Autodesk Inventor part; units mm, degrees
ref_plane "YZ Plane" through (0, 0, 0) normal (1, 0, 0) x (0, 1, 0)
ref_plane "XZ Plane" through (0, 0, 0) normal (0, 1, 0) x (-1, 0, 0)
ref_plane "XY Plane" through (0, 0, 0) normal (0, 0, 1) x (1, 0, 0)
sketch "Sketch1" plane through (0, 0, 0) normal (0, 1, 0) x (-1, 0, 0)
  line L0 (0, 0) -> (45, 0)
  line L1 (45, 0) -> (14.87, 0)
  line L2 (14.87, -170.18) -> (56.523, -170.18)
  line L3 (144.78, -163.83) -> (144.78, -85.18)
  line L4 (144.78, -85.18) -> (45, -85.18)
  line L5 (144.78, -163.83) -> (144.78, -170.18)
  line L6 (113.657, -170.18) -> (144.78, -170.18)
  line L7 (144.78, -170.18) -> (0, -170.18)
  line L8 (45, 0) -> (45, -85.18)
  circle A0 centre (5.08, -6.35) radius 1.75
  circle A1 centre (5.08, -163.83) radius 1.75
  circle A2 centre (137.16, -163.83) radius 1.75
  circle A3 centre (83.48, -93.35) radius 1.75
  circle A4 centre (83.48, -156.35) radius 1.75
  line L9 (-36.027, -96.0808) -> (-36.027, -97.5854)
  line L10 (-39.0316, -99.0854) -> (-39.0316, -71.0946)
  line L11 (-8.0362, -74.0992) -> (-8.0362, -72.5946)
  line L12 (-8.0362, -72.5946) -> (-8.0362, -74.0992)
  line L13 (-36.027, -68.09) -> (-8.0362, -68.09)
  arc A5 (-36.027, -96.0808) -> (-39.0316, -99.0854) centre (-36.027, -99.0854) ccw
  arc A6 (-8.0362, -68.09) -> (-11.0408, -71.0946) centre (-8.0362, -71.0946) ccw
  arc A7 (-36.027, -97.5854) -> (-34.527, -99.0854) centre (-36.027, -99.0854) ccw
  arc A8 (-36.027, -97.5854) -> (-34.527, -99.0854) centre (-36.027, -99.0854) ccw
  arc A9 (-8.0362, -72.5946) -> (-9.5362, -71.0946) centre (-8.0362, -71.0946) ccw
  arc A10 (-8.0362, -72.5946) -> (-9.5362, -71.0946) centre (-8.0362, -71.0946) ccw
  arc A11 (-8.0362, -74.0992) -> (-5.0316, -71.0946) centre (-8.0362, -71.0946) ccw
  line L14 (-5.0316, -99.0854) -> (-5.0316, -71.0946)
  line L15 (-8.0362, -102.09) -> (-36.027, -102.09)
  line L16 (-36.027, -102.09) -> (-8.0362, -102.09)
  arc A12 (-9.5362, -99.0854) -> (-8.0362, -97.5854) centre (-8.0362, -99.0854) ccw
  arc A13 (-9.5362, -99.0854) -> (-8.0362, -97.5854) centre (-8.0362, -99.0854) ccw
  arc A14 (-34.527, -71.0946) -> (-36.027, -72.5946) centre (-36.027, -71.0946) ccw
  arc A15 (-34.527, -71.0946) -> (-36.027, -72.5946) centre (-36.027, -71.0946) ccw
  line L17 (-8.0362, -97.5854) -> (-8.0362, -96.0808)
  arc A16 (-5.0316, -99.0854) -> (-8.0362, -96.0808) centre (-8.0362, -99.0854) ccw
  arc A17 (-5.0316, -99.0854) -> (-8.0362, -96.0808) centre (-8.0362, -99.0854) ccw
  line L18 (-8.0362, -97.5854) -> (-8.0362, -96.0808)
  line L19 (-34.527, -71.0946) -> (-33.0224, -71.0946)
  arc A18 (-33.0224, -71.0946) -> (-36.027, -68.09) centre (-36.027, -71.0946) ccw
  arc A19 (-39.0316, -71.0946) -> (-36.027, -74.0992) centre (-36.027, -71.0946) ccw
  arc A20 (-39.0316, -71.0946) -> (-36.027, -74.0992) centre (-36.027, -71.0946) ccw
  arc A21 (-33.0224, -71.0946) -> (-36.027, -68.09) centre (-36.027, -71.0946) ccw
  line L20 (-11.0408, -71.0946) -> (-9.5362, -71.0946)
  line L21 (-9.5362, -71.0946) -> (-11.0408, -71.0946)
  line L22 (-36.027, -97.5854) -> (-36.027, -96.0808)
  arc A22 (-36.027, -96.0808) -> (-39.0316, -99.0854) centre (-36.027, -99.0854) ccw
  line L23 (-34.527, -99.0854) -> (-33.0224, -99.0854)
  line L24 (-34.527, -99.0854) -> (-33.0224, -99.0854)
  arc A23 (-36.027, -102.09) -> (-33.0224, -99.0854) centre (-36.027, -99.0854) ccw
  line L25 (-11.0408, -99.0854) -> (-9.5362, -99.0854)
  line L26 (-11.0408, -99.0854) -> (-9.5362, -99.0854)
  arc A24 (-11.0408, -99.0854) -> (-8.0362, -102.09) centre (-8.0362, -99.0854) ccw
  line L27 (-36.027, -74.0992) -> (-36.027, -72.5946)
  line L28 (-36.027, -72.5946) -> (-36.027, -74.0992)
  line L29 (-36.027, -99.0854) -> (-23.327, -99.0854) construction
  line L30 (-36.027, -99.0854) -> (-27.137, -99.0854) construction
  arc A25 (-44.0632, -105.3716) -> (-42.3132, -107.1216) centre (-42.3132, -105.3716) ccw
  arc A26 (-42.3132, -63.0584) -> (-44.0632, -64.8084) centre (-42.3132, -64.8084) ccw
  line L31 (-42.3132, -63.0584) -> (0, -63.0584)
  line L32 (0, -107.1216) -> (-42.3132, -107.1216)
  line L33 (-44.0632, -105.3716) -> (-44.0632, -64.8084)
  line L34 (0, -170.18) -> (0, -107.1216)
  line L35 (0, -63.0584) -> (0, 0)
  circle A27 centre (10.16, -127.8558) radius 1.5
  circle A28 centre (10.16, -149.4458) radius 1.5
  circle A29 centre (25.4, -149.4458) radius 1.5
  circle A30 centre (25.4, -127.8558) radius 1.4986
  point P0 (-2.54, 0.1)
  dimension "d3" = 3.5
  dimension "d5" = 3.5
  dimension "d6" = 3.5
  dimension "d9" = 3
  dimension "d10" = 3
  dimension "d11" = 3
  dimension "d12" = 2.9972
extrude "Extrusion1" add sketch "Sketch1" along normal blind 2.286
fillet "Fillet1" radius 3.175 8 edges at (-45, 1.143, 0) (0, 1.143, 0) (0, 1.143, -63.0584) (0, 1.143, -107.1216) (-45, 1.143, -85.18) (-144.78, 1.143, -85.18) (-144.78, 1.143, -170.18) (0, 1.143, -170.18)
sketch "Sketch2" plane through (0, 2.286, 0) normal (0, 1, 0) x (1, 0, 0)
  circle A0 centre (-51.7938, 156.5362) radius 1.75
  circle A1 centre (-115.1662, 156.5362) radius 1.75
  circle A2 centre (-115.1662, 93.1638) radius 1.65
  circle A3 centre (-115.1662, 93.1638) radius 1.75
  circle A4 centre (-51.7938, 93.1638) radius 1.65
  circle A5 centre (-51.7938, 93.1638) radius 1.75
  line L0 (-144.78, 167.005) -> (-144.78, 88.355)
  line L1 (0, 110.2966) -> (0, 167.005)
  circle A6 centre (-83.48, 93.35) radius 1.75
  circle A7 centre (-83.48, 156.35) radius 1.75
  point P0 (0, 0)
  dimension "d17" = 3.5
  dimension "d18" = 3.5
  dimension "d19" = 3.5
  dimension "d20" = 3.5
extrude "Extrusion2" cut sketch "Sketch2" against normal blind 25.4 contours A0 | A1 | A2 | A3 | A4 | A5
sketch "Sketch3" plane through (0, 2.286, 0) normal (0, 1, 0) x (1, 0, 0)
  circle A0 centre (-5.08, 6.35) radius 1.75
  arc A1 (-17.78, 9.525) -> (-11.43, 9.525) centre (-14.605, 9.525) ccw
  arc A2 (-30.48, 9.525) -> (-24.13, 9.525) centre (-27.305, 9.525) ccw
  arc A3 (-11.43, 73.025) -> (-17.78, 73.025) centre (-14.605, 73.025) ccw
  arc A4 (-24.13, 98.425) -> (-30.48, 98.425) centre (-27.305, 98.425) ccw
  line L0 (-30.48, 9.525) -> (-30.48, 98.425)
  line L1 (-24.13, 98.425) -> (-24.13, 9.525)
  line L2 (-17.78, 9.525) -> (-17.78, 73.025)
  line L3 (-11.43, 73.025) -> (-11.43, 9.525)
  point P0 (0, 0)
extrude "Extrusion3" cut sketch "Sketch3" against normal blind 25.4 contours L2 A3 L3 A1 | L0 A4 L1 A2
sketch "Sketch4" plane through (0, 2.286, 0) normal (0, 1, 0) x (1, 0, 0)
  circle A0 centre (-5.08, 6.35) radius 1.75
  circle A1 centre (-5.08, 6.35) radius 1.75
  arc A2 (-5.08, 11.43) -> (-5.08, 1.27) centre (-5.08, 6.35) ccw
  line L0 (0, 3.175) -> (0, 59.8834)
  line L1 (-5.08, 1.27) -> (5.0316, 1.27)
  line L2 (5.0316, 1.27) -> (5.0316, 63.0584)
  line L3 (-5.08, 11.43) -> (0, 11.43)
  line L4 (0, 11.43) -> (0, 59.8834)
  line L5 (3.175, 63.0584) -> (42.3132, 63.0584)
  line L6 (5.0316, 63.0584) -> (42.3132, 63.0584)
  line L7 (44.0632, 64.8084) -> (44.0632, 105.3716)
  line L8 (44.0632, 64.8084) -> (44.0632, 105.3716)
  line L9 (42.3132, 107.1216) -> (3.175, 107.1216)
  line L10 (42.3132, 107.1216) -> (5.0316, 107.1216)
  line L11 (5.0316, 107.1216) -> (5.0316, 170.18)
  circle A3 centre (-5.08, 163.83) radius 1.75
  circle A4 centre (-5.08, 163.83) radius 1.75
  circle A5 centre (-5.08, 163.83) radius 5.08
  line L12 (0, 110.2966) -> (0, 167.005)
  line L13 (-5.08, 168.91) -> (5.0316, 168.91)
  line L14 (0, 59.8834) -> (0, 158.75)
  line L15 (0, 158.75) -> (-5.08, 158.75)
  arc A6 (8.0362, 72.5946) -> (9.5362, 71.0946) centre (8.0362, 71.0946) ccw
  arc A7 (8.0362, 72.5946) -> (9.5362, 71.0946) centre (8.0362, 71.0946) ccw
  arc A8 (34.527, 71.0946) -> (36.027, 72.5946) centre (36.027, 71.0946) ccw
  arc A9 (34.527, 71.0946) -> (36.027, 72.5946) centre (36.027, 71.0946) ccw
  arc A10 (36.027, 97.5854) -> (34.527, 99.0854) centre (36.027, 99.0854) ccw
  arc A11 (36.027, 97.5854) -> (34.527, 99.0854) centre (36.027, 99.0854) ccw
  arc A12 (9.5362, 99.0854) -> (8.0362, 97.5854) centre (8.0362, 99.0854) ccw
  arc A13 (9.5362, 99.0854) -> (8.0362, 97.5854) centre (8.0362, 99.0854) ccw
  arc A14 (8.0362, 68.09) -> (11.0408, 71.0946) centre (8.0362, 71.0946) ccw
  arc A15 (33.0224, 71.0946) -> (36.027, 68.09) centre (36.027, 71.0946) ccw
  line L16 (11.0408, 99.0854) -> (9.5362, 99.0854)
  line L17 (36.027, 68.09) -> (8.0362, 68.09)
  line L18 (8.0362, 68.09) -> (36.027, 68.09)
  line L19 (5.0316, 99.0854) -> (5.0316, 71.0946)
  line L20 (5.0316, 71.0946) -> (5.0316, 99.0854)
  line L21 (8.0362, 102.09) -> (36.027, 102.09)
  line L22 (8.0362, 102.09) -> (36.027, 102.09)
  line L23 (39.0316, 71.0946) -> (39.0316, 99.0854)
  line L24 (39.0316, 71.0946) -> (39.0316, 99.0854)
  line L25 (33.0224, 71.0946) -> (34.527, 71.0946)
  line L26 (34.527, 71.0946) -> (33.0224, 71.0946)
  line L27 (36.027, 72.5946) -> (36.027, 74.0992)
  line L28 (36.027, 72.5946) -> (36.027, 74.0992)
  line L29 (9.5362, 71.0946) -> (11.0408, 71.0946)
  line L30 (11.0408, 71.0946) -> (9.5362, 71.0946)
  line L31 (8.0362, 74.0992) -> (8.0362, 72.5946)
  line L32 (8.0362, 72.5946) -> (8.0362, 74.0992)
  line L33 (8.0362, 96.0808) -> (8.0362, 97.5854)
  line L34 (8.0362, 96.0808) -> (8.0362, 97.5854)
  arc A16 (11.0408, 99.0854) -> (8.0362, 102.09) centre (8.0362, 99.0854) ccw
  line L35 (9.5362, 99.0854) -> (11.0408, 99.0854)
  line L36 (36.027, 97.5854) -> (36.027, 96.0808)
  line L37 (36.027, 96.0808) -> (36.027, 97.5854)
  line L38 (33.0224, 99.0854) -> (34.527, 99.0854)
  line L39 (34.527, 99.0854) -> (33.0224, 99.0854)
  arc A17 (36.027, 96.0808) -> (39.0316, 99.0854) centre (36.027, 99.0854) ccw
  arc A18 (36.027, 102.09) -> (33.0224, 99.0854) centre (36.027, 99.0854) ccw
  arc A19 (33.0224, 71.0946) -> (36.027, 68.09) centre (36.027, 71.0946) ccw
  arc A20 (39.0316, 71.0946) -> (36.027, 74.0992) centre (36.027, 71.0946) ccw
  arc A21 (8.0362, 68.09) -> (11.0408, 71.0946) centre (8.0362, 71.0946) ccw
  arc A22 (8.0362, 74.0992) -> (5.0316, 71.0946) centre (8.0362, 71.0946) ccw
  arc A23 (11.0408, 99.0854) -> (8.0362, 102.09) centre (8.0362, 99.0854) ccw
  arc A24 (5.0316, 99.0854) -> (8.0362, 96.0808) centre (8.0362, 99.0854) ccw
  point P0 (0, 0)
  point P1 (3.175, 59.8834)
properties part number "ThirdLayer"
The listing builds one solid part. Answer for the finished solid, in the listing's coordinates (mm). Round coordinates to 2 decimals unless told otherwise and drop trailing zeros. Loops run counter-clockwise (first coordinate to the right, second up) from the corner with the lowest first, then second, coordinate; pieces in that order, holes last. Notation, with made-up numbers: M 88.25,-13.75 L 108.25,-13.75 A29 cw 108.25,10.25 Z; hole C 17,42 d11. An arc over 180 degrees is marked long. Write each question's results on one line, items separated by ' | '. Start each with the question number.
1) Find section A-A on z = -44. Write down the section's boundary in (x, y), plus the area to 3 significant figures.
2) Find section B-B on x = -90. Write down the section's boundary in (y, z).
3) Find section D-D on z = -142. Write down the section's boundary in (x, y).
4) Each of these flat-tipped pins is pushed along its axis until it touches: pin 1 (1.8 mm diameter, centred on x = -25.4, z = -149.45, fed in from +Y); pin 2 (1.2 mm diameter, centred on x = 10, y = 1, fed in from -Z); pin 3 (1.1 mm diameter, centred on x = 21, y = 1.5, fed in from +Z); pin 4 (0.7 mm diameter, centred on y = 1, z = -44.5, fed in from -X). Where does it stop, or does it pass through?
5) Find section C-C on y = 1.5. Count the separate pieces of the cut face and the enclosed holes in it, plus the area to 3 significant figures.
6) Straight lines are drawn through the part: probe 1 along X at (y, z) = (0.7, -163.83); probe 2 along X at (y, z) = (1.4, -22.5); probe 3 along Z at (x, y) = (-116, 1.35). For each, find the intervals that lie inside material, in ascending order.
Final values:
1) outline: M -45,0 L -30.48,0 L -30.48,2.29 L -45,2.29 Z; M -24.13,0 L -17.78,0 L -17.78,2.29 L -24.13,2.29 Z; M -11.43,0 L 0,0 L 0,2.29 L -11.43,2.29 Z | area: 73.8 mm²
2) outline: M 0,-170.18 L 2.29,-170.18 L 2.29,-85.18 L 0,-85.18 Z
3) outline: M -144.78,0 L 0,0 L 0,2.29 L -144.78,2.29 Z
4) pin 1: through | pin 2: z = -107.12 | pin 3: z = -63.06 | pin 4: x = -45
5) separate pieces: 1 | enclosed holes: 16 | area: 15,800 mm²
6) probe 1: -144.78 to -138.91, -135.41 to -6.83, -3.33 to 0 | probe 2: -45 to -30.48, -24.13 to -17.78, -11.43 to 0 | probe 3: -170.18 to -158.07, -155 to -94.7, -91.63 to -85.18
